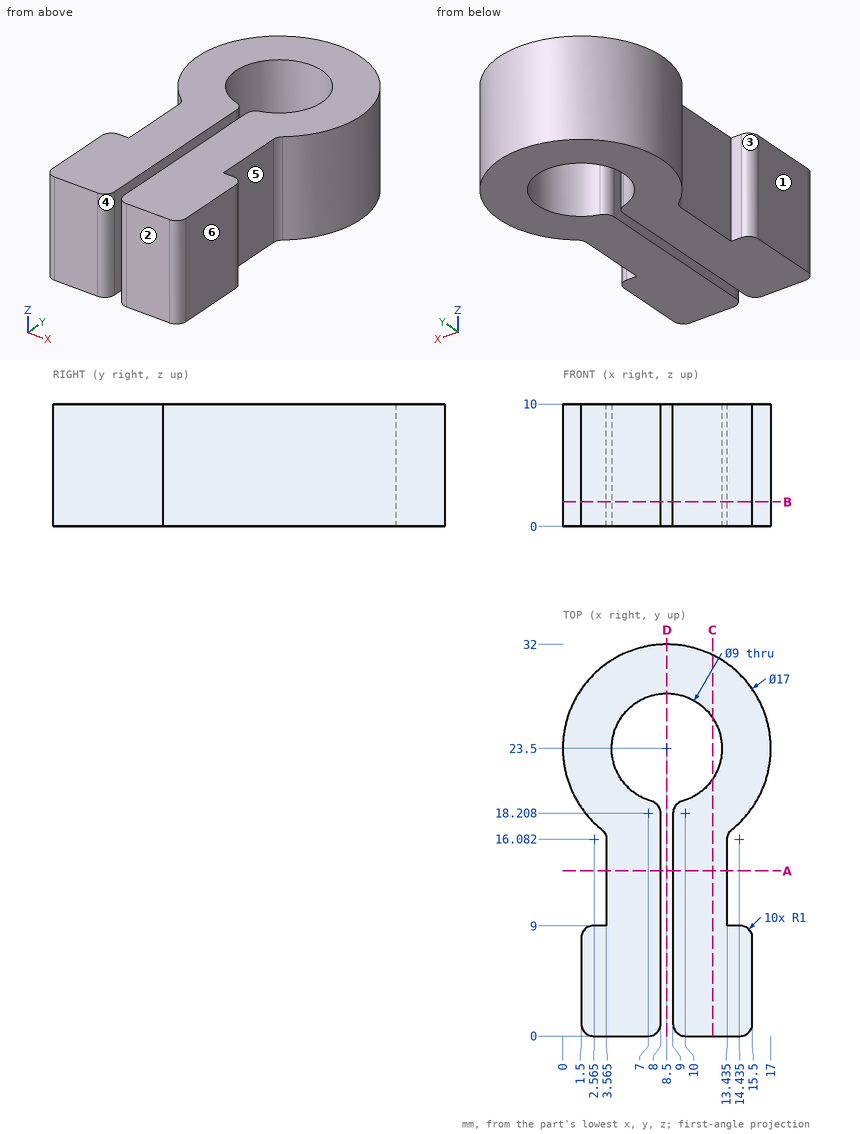
Input: dimensioned drawing with shaded views. Units: mm. Origin: part minimum x, y, z. A direction names the side the tool comes from. Give positions to 0.01 mm unless a question says otherwise; leave off trailing zeros. Loops run counter-clockwise (first coordinate to the right, second up) from the corner with the lowest first, then second, coordinate; pieces in that order, holes last. Notation, with made-up numbers: (11.25, 30) -> (56.25, 30) arc R23 cw to (56.25, 50) -> close; hole circle Ø5 at (9.5, 28). An arc over 180 degrees is marked (long way). Return JSON: item names as keys, results as strings.
Item 1: Line query: line 1 (X direction, y = 7, z = 8); line 2 (X direction, y = 16, z = 7.5) (1 decimal); line 3 (Y direction, x = 8.5, z = 2.25). Output: solid intervals per line, ascending.
Filled in:
{"line 1": "1.5 to 8, 9 to 15.5", "line 2": "3.6 to 8, 9 to 13.4", "line 3": "28 to 32"}
Item 2: Mould query, pull axis Y, two halves, no side actions, for the marked faces 4, 5 and 6. Classes: released by +Y, released by -Y, zero draft, split by the parting line, or undercut.
Filled in:
{"face 4": "released by -Y", "face 5": "undercut", "face 6": "zero draft"}
Item 3: Section A-A, the plane y = 13.5. Output: boundary loops of the cut face in (x, z) (1 decimal).
Filled in:
{"outline": "(3.6, 0) -> (8, 0) -> (8, 10) -> (3.6, 10) -> close; (9, 0) -> (13.4, 0) -> (13.4, 10) -> (9, 10) -> close"}
Item 4: Section D-D, the plane x = 8.5. Output: boundary loops of the cut face in (y, z).
Filled in:
{"outline": "(28, 0) -> (32, 0) -> (32, 10) -> (28, 10) -> close"}
Item 5: Section B-B, the plane z = 2. Output: boundary loops of the cut face in (x, y) (1 decimal).
Filled in:
{"outline": "(1.5, 1) arc R1 ccw to (2.5, 0) -> (7, 0) arc R1 ccw to (8, 1) -> (8, 18.2) arc R1 ccw to (7.3, 19.2) arc R4.5 cw (long way) to (9.7, 19.2) arc R1 ccw to (9, 18.2) -> (9, 1) arc R1 ccw to (10, 0) -> (14.5, 0) arc R1 ccw to (15.5, 1) -> (15.5, 8) arc R1 ccw to (14.5, 9) -> (13.4, 9) -> (13.4, 16.1) arc R1 cw to (13.8, 16.9) arc R8.5 ccw (long way) to (3.2, 16.9) arc R1 cw to (3.6, 16.1) -> (3.6, 9) -> (2.5, 9) arc R1 ccw to (1.5, 8) -> close"}
Item 6: Access query for the marked faces 1, 2 and 3. Directions: +Z, -Z, +X, -X, +Y, -Y. A direction counts if a zero-diameter tool reaches every point of the face in a straight line with its end or side. Return the directions, or none.
Filled in:
{"face 1": "+Z, -Z, -X, -Y", "face 2": "+Z, -Z, +X, -X, -Y", "face 3": "+Z, -Z, -X"}
Item 7: Pin query (flat end, axial travel): P1, Ø1.5, axis at x = 6, z = 3, coming from the +Y side; P2, Ø5.5, axis at y = 4, z = 4.5, coming from the +X side; P3, Ø4, axis at x = 13.5, z = 6.5, coming from the +Y side. Return the tip coordinate at first contact, or that it passes through.
Filled in:
{"P1": "y = 31.82", "P2": "x = 15.5", "P3": "y = 31.45"}
Item 8: Section C-C, the plane x = 12.25. Output: boundary loops of the cut face in (y, z).
Filled in:
{"outline": "(0, 0) -> (21.01, 0) -> (21.01, 10) -> (0, 10) -> close; (25.99, 0) -> (31.13, 0) -> (31.13, 10) -> (25.99, 10) -> close"}
